Can you work these out from the model? Positions are in its coordinate system, mm. A direction names the side the tool comes from. Coordinates: 2 decimals unless noted, no trailing zeros. Order: outer loops, then holes, each group sorted by start corner. A loop starts at its lowest first (then second) coordinate and runs counter-clockwise, first axis right, second up. Notation, with made-up numbers: (15.5, 52) -> (37.5, 52) arc R29 ccw to (37.5, 79) -> close; hole circle Ø4 at (-6.5, 34). An arc over 180 degrees is marked (long way). Answer in a Markdown table with one row per item.
```python
from build123d import *

# Parameters (mm, degrees)
SKETCH1_R           = 1.5
BOSS_EXTRUDE1_DEPTH = 1.524


with BuildPart() as part:
    # Sketch1 → Boss-Extrude1 (new body)
    with BuildSketch(Plane(origin=(0, 0, 0), x_dir=(1, 0, 0), z_dir=(0, 1, 0))):
        with BuildLine():
            Line((14.035300806, 5.461735825), (21.10663358, 5.652076803))
            ThreePointArc((21.10663358, 5.652076803), (21.913592667, 5.50842857), (22.59815065, 5.057653515))
            Line((22.59815065, 5.057653515), (22.609206424, 5.046597741))
            ThreePointArc((22.609206424, 5.046597741), (23.038239741, 4.414453667), (23.203514475, 3.668558246))
            ThreePointArc((23.203514475, 3.668558246), (29.19167252, 1.17868297), (27.085559617, 7.312344528))
            ThreePointArc((27.085559617, 7.312344528), (26.071299756, 7.588172266), (25.211041867, 8.192126215))
            Line((25.211041867, 8.192126215), (25.162863778, 8.240304305))
            ThreePointArc((25.162863778, 8.240304305), (23.45146882, 9.367241942), (21.434071104, 9.726362525))
            Line((21.434071104, 9.726362525), (13.521182629, 9.513369165))
            ThreePointArc((13.521182629, 9.513369165), (11.650868629, 9.101934762), (10.065770406, 8.027310944))
            Line((10.065770406, 8.027310944), (9.730613659, 7.692154197))
            ThreePointArc((9.730613659, 7.692154197), (8.87035577, 7.088200248), (7.856095909, 6.81237251))
            ThreePointArc((7.856095909, 6.81237251), (5.749983006, 0.678710952), (11.738141051, 3.168586228))
            ThreePointArc((11.738141051, 3.168586228), (11.903415785, 3.914481649), (12.332449102, 4.546625723))
            Line((12.332449102, 4.546625723), (12.653135916, 4.867312537))
            ThreePointArc((12.653135916, 4.867312537), (13.287175206, 5.297162064), (14.035300806, 5.461735825))
        make_face()
        with Locations(Location((8.183630247, 3.271488826, 0), (0, 0, 90))):
            Circle(SKETCH1_R, mode=Mode.SUBTRACT)
        with Locations(Location((26.758025279, 3.771460844, 0), (0, 0, 90))):
            Circle(SKETCH1_R, mode=Mode.SUBTRACT)
    extrude(amount=BOSS_EXTRUDE1_DEPTH)


solid = part.part
```
(1) We'd pull the mould along X, two halves only. Please class faces 3 (the flat face through (17, 0, -6)), 4 (the cylindrical face through (5.668, 0.751, -0.758)), 5 (the cylindrical face through (11.676, 0.751, -9.113)): +X half, -X half, draft (parallel to the pull), parting line (faces both ways), or undercut.
Response values:
| item | result |
|---|---|
| face 3 | draft |
| face 4 | undercut |
| face 5 | -X half |
(2) On a 3-axis mill with a long thin cutter (end or side, diameter ignored), from which of +Z, -Z, +X, -X, +Y, -Y can I reach the whole of each face in a straight line? I mean faces 1 (the cylindrical face through (8.884, 0.751, -7.095)), 2 (the cylindrical face through (13.277, 0.751, -5.293)). Say none if no direction works.
Response values:
| item | result |
|---|---|
| face 1 | -Z, -X, +Y, -Y |
| face 2 | +Z, +Y, -Y |
(3) Will this pin go through, and if not, where does the flat tip stop? pin 1 Ø5 at (x, z) = (8.18, -3.27) entering from +Y.
Response values:
| item | result |
|---|---|
| pin 1 | y = 1.52 |
(4) Suppose I cut it at A-A (z = -0.5). Please give me the cut outline in (x, y), and give its area (3 significant figures).
Response values:
| item | result |
|---|---|
| outline | (5.96, 0) -> (10.41, 0) -> (10.41, 1.52) -> (5.96, 1.52) -> close; (25.36, 0) -> (28.15, 0) -> (28.15, 1.52) -> (25.36, 1.52) -> close |
| area | 11.0 mm2 |
(5) I need wall thicknesses on line 1 (X direction, y = 0.95, z = -3.5); line 2 (X direction, y = 0.25, z = -3.25); line 3 (Z direction, x = 27, y = 1.4). Which ranges of each line are inside material? Lowest first, please. Write a range as [from, to].
Response values:
| item | result |
|---|---|
| line 1 | [4.63, 6.7], [9.67, 11.78], [23.21, 25.28], [28.23, 30.3] |
| line 2 | [4.63, 6.68], [9.68, 11.74], [23.24, 25.35], [28.16, 30.28] |
| line 3 | [-7.32, -5.25], [-2.29, -0.22] |
(6) Suppose I cut it at C-C (x = 17.75). Please give me the cut outline in (y, z).
Response values:
| item | result |
|---|---|
| outline | (0, -9.63) -> (1.52, -9.63) -> (1.52, -5.56) -> (0, -5.56) -> close |
(7) Suppose I cut it at B-B (y = 0.9). Count the separate pieces of the cut face and the enclosed holes in it, and give its area (3 significant figures).
Response values:
| item | result |
|---|---|
| separate pieces | 1 |
| enclosed holes | 2 |
| area | 127 mm2 |
(8) Suppose I cut it at D-D (z = -8.5). Please give me the cut outline in (x, y), and give its area (3 significant figures).
Response values:
| item | result |
|---|---|
| outline | (10.61, 0) -> (24.88, 0) -> (24.88, 1.52) -> (10.61, 1.52) -> close |
| area | 21.8 mm2 |
